Geometry: final body of the model. Coordinates: model frame, mm. Give positions to 0.01 mm unless a question says otherwise; leave off trailing zeros. Write each loop counter-clockwise with the first axis right and the second up, starting at its lowest first coordinate (ties: lowest second). Pieces come first, ordered by that corner, then holes. Notation, with made-up numbers: (89.25, 85) -> (131.25, 85) arc R13 cw to (131.25, 91) -> close; hole circle Ø1 at (3, 83). An arc over 180 degrees is marked (long way). Answer as a JSON object with one key per item and string values.
from build123d import *

# Parameters (mm, degrees)
F0_R     = 4
F1_DEPTH = 3


# Not quite as in the source:
# - a feature names something its author has since deleted; it is built from what else it names


with BuildPart() as f1:
    # F0 (on Top) → F1 (new body)
    with BuildSketch(Plane.XY):
        with BuildLine():
            Line((-11.4797556719, -12.5), (-47.2819722649, -134.6362324887))
            ThreePointArc((-47.2819722649, -134.6362324887), (-46.6657765426, -140.3433149262), (-42.1945436765, -143.9431154447))
            ThreePointArc((-42.1945436765, -143.9431154447), (-36.487461239, -143.3269197224), (-32.8876607204, -138.8556868563))
            Line((-32.8876607204, -138.8556868563), (4.0370171151, -12.8902728162))
            Line((4.0370171151, -12.8902728162), (5.6170864437, -7.5))
            Line((5.6170864437, -7.5), (-10.0140883648, -7.5))
            Line((-10.0140883648, -7.5), (-11.4797556719, -12.5))
        make_face()
        with Locations((-40.0848164926, -136.7459596725)):
            Circle(F0_R, mode=Mode.SUBTRACT)
    extrude(amount=F1_DEPTH)


solid = f1.part
Q1. Material intervals for L1, parallel to X at y = -31, z = 1.9; L2, parallel to X at y = -96, z = 1.2, sorted ascending. Write a range as from..to.
Values:
{"L1": "-16.9..-1.27", "L2": "-35.96..-20.33"}
Q2. Cut plane B-B (z = 2.55). Return the cut outline in (x, y), and give its area (3 significant figures).
Values:
{"outline": "(-47.28, -134.64) arc R7.5 ccw to (-32.89, -138.86) -> (5.62, -7.5) -> (-10.01, -7.5) -> close; hole circle Ø8 at (-40.08, -136.75)", "area": "2,060 mm²"}
Q3. Cut plane C-C (y = -106.5). Return the cut outline in (x, z).
Values:
{"outline": "(-39.03, 0) -> (-23.4, 0) -> (-23.4, 3) -> (-39.03, 3) -> close"}
Q4. Cut plane D-D (x = 0). Return the cut outline in (y, z).
Values:
{"outline": "(-26.66, 0) -> (-7.5, 0) -> (-7.5, 3) -> (-26.66, 3) -> close"}
Q5. First-contact query: P1, Ø6.5, axis at x = -40.08, y = -136.75, coming from the -Z side; P2, Ø1.5, axis at y = -30.5, z = 1, coming from the -X side. Flat tips, straight axial feed; report the tip coordinate or a pass-through.
Values:
{"P1": "through", "P2": "x = -16.98"}
Q6. Cut plane A-A (x = -38). Return the cut outline in (y, z), and give its area (3 significant figures).
Values:
{"outline": "(-143.95, 0) -> (-140.16, 0) -> (-140.16, 3) -> (-143.95, 3) -> close; (-133.33, 0) -> (-102.97, 0) -> (-102.97, 3) -> (-133.33, 3) -> close", "area": "102 mm²"}
Q7. Mould query, pull axis Y, two halves, no side actions, for faces 1 (the flat face through (-21, -76, 0)), 2 (the cylindrical face through (-43.03, -134.04, 1.48)), 3 (the flat face through (-2, -7.5, 1)). Classes: pulls with the +Y half, pulls with the -Y half, needs draft (parallel to the pull), parting line crosses it, or undercut.
Values:
{"face 1": "needs draft", "face 2": "undercut", "face 3": "pulls with the +Y half"}
